Verification items for this drawing (mm, ordinates from the low corner). Round coordinates to 2 decimals unless told otherwise and drop trailing zeros. Loops run counter-clockwise (first coordinate to the right, second up) from the corner with the lowest first, then second, coordinate; pieces in that order, holes last. Notation, with made-up numbers: M -36,12 L -28,12 A33 ccw -28,48 Z; hole C -23,-34.75 d1. An arc over 180 degrees is marked long. Write item = value, one per line.
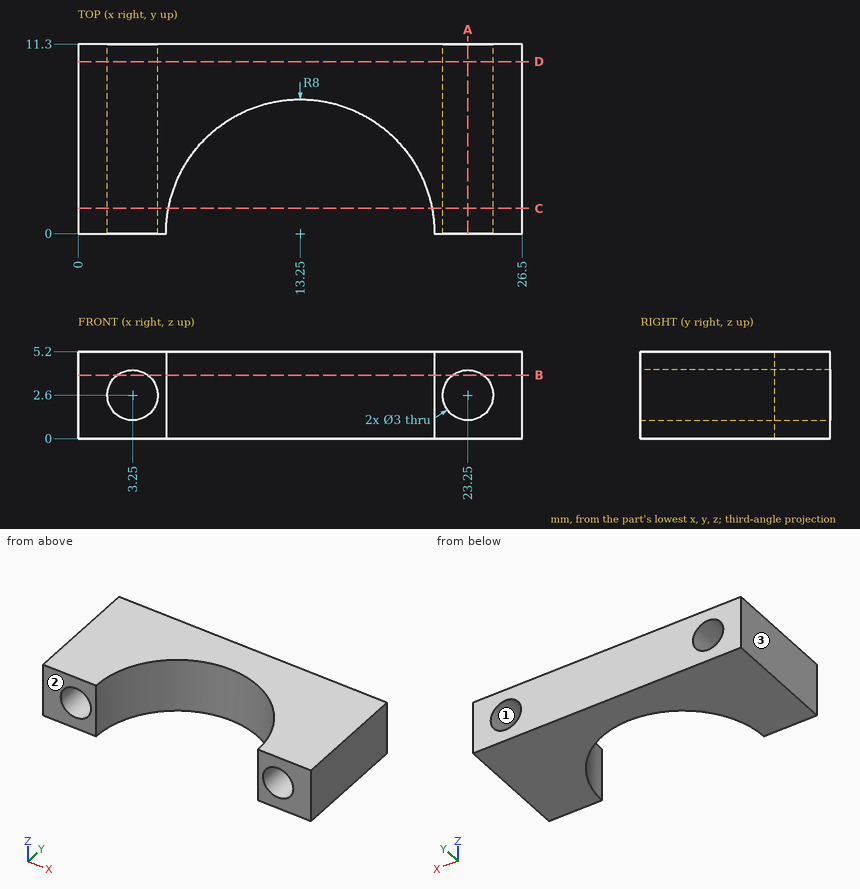
(1) Sectioned sample at D-D on y = 10.25. Record the cut outline in (x, z), then the cut area to 3 significant figures.
Result set:
outline = M 0,0 L 26.5,0 L 26.5,5.2 L 0,5.2 Z; hole C 3.25,2.6 d3; hole C 23.25,2.6 d3
area = 124 mm2
(2) Release check for a two-part mould opening along X. For the marked faces 1, 2 and 3 record: released by +X, released by -X, zero draft, split by the parting line, or undercut.
Result set:
face_1 = undercut
face_2 = zero draft
face_3 = released by -X
(3) Sectioned sample at C-C on y = 1.5. Record the cut outline in (x, z).
Result set:
outline = M 0,0 L 5.39,0 L 5.39,5.2 L 0,5.2 Z; M 21.11,0 L 26.5,0 L 26.5,5.2 L 21.11,5.2 Z; hole C 3.25,2.6 d3; hole C 23.25,2.6 d3
(4) Material ranges on line 1 along X through (y, z) = (4, 3.6); line 2 along X through (y, z) = (6.5, 2.6); line 3 along X through (y, z) = (10, 2.85), recorded low to high. Write a range as from..to.
Result set:
line_1 = 0..2.13, 4.37..6.32, 20.18..22.13, 24.37..26.5
line_2 = 0..1.75, 4.75..8.59, 17.91..21.75, 24.75..26.5
line_3 = 0..1.77, 4.73..21.77, 24.73..26.5
(5) Sectioned sample at A-A on x = 23.25. Record the cut outline in (y, z), then the cut area to 3 significant figures.
Result set:
outline = M 0,0 L 11.3,0 L 11.3,1.1 L 0,1.1 Z; M 0,4.1 L 11.3,4.1 L 11.3,5.2 L 0,5.2 Z
area = 24.9 mm2
(6) Sectioned sample at B-B on z = 3.8. Record the cut outline in (x, y), then the cut area to 3 significant figures.
Result set:
outline = M 0,0 L 2.35,0 L 2.35,11.3 L 0,11.3 Z; M 4.15,0 L 5.25,0 A8 cw 21.25,0 L 22.35,0 L 22.35,11.3 L 4.15,11.3 Z; M 24.15,0 L 26.5,0 L 26.5,11.3 L 24.15,11.3 Z
area = 158 mm2
